```python
from build123d import *

# Parameters (mm, degrees)
SKETCH1_W                  = 38.1
SKETCH1_H                  = 4.365625
BOSS_EXTRUDE1_DEPTH        = 12.7
BOSS_EXTRUDE3_DEPTH        = 12.7
SKETCH8_R                  = 2.1828125
CUT_EXTRUDE1_DEPTH         = 30.170285502
SKETCH11_R                 = 2.1828125
CUT_EXTRUDE2_DEPTH         = 30.170285502
FILLET1_R                  = 3.175
FILLET2_R                  = 3.175
F_4_40_TAPPED_HOLE1_D      = 2.2606
BOSS_EXTRUDE4_DEPTH        = 12.7
TAP_DRILL_FOR_10_32_TAP1_D = 4.0386
FILLET3_R                  = 1.27
FILLET4_R                  = 1.27
CHAMFER1_SIZE              = 0.254


with BuildPart() as part:
    # Sketch1 → Boss-Extrude1 (new body)
    with BuildSketch(Plane.XY):
        Polygon((6.35, 5.08), (25.4, 5.08), (25.4, -5.08), (-25.4, -5.08), (-25.4, 5.08), (-6.35, 5.08), align=None)
        Rectangle(SKETCH1_W, SKETCH1_H, mode=Mode.SUBTRACT)
    extrude(amount=BOSS_EXTRUDE1_DEPTH)

    # Sketch7 → Boss-Extrude3 (add)
    with BuildSketch(Plane.XY.offset(12.7)):
        with BuildLine():
            Line((-20.290450061, 5.08), (-13.443924939, 5.08))
            ThreePointArc((-13.443924939, 5.08), (-16.8671875, 6.6675), (-20.290450061, 5.08))
        make_face()
    boss_extrude3 = extrude(amount=-BOSS_EXTRUDE3_DEPTH)

    # Sketch8 → Cut-Extrude1 (cut, through all)
    with BuildSketch(Plane.XY.offset(12.7)):
        with Locations((-16.8671875, 2.1828125)):
            Circle(SKETCH8_R)
    cut_extrude1 = extrude(amount=-CUT_EXTRUDE1_DEPTH, mode=Mode.SUBTRACT)

    # Sketch11 → Cut-Extrude2 (cut, through all)
    with BuildSketch(Plane.XY.offset(12.7)):
        with Locations((-17.159628923, -1.09140625)):
            Circle(SKETCH11_R)
    cut_extrude2 = extrude(amount=-CUT_EXTRUDE2_DEPTH, mode=Mode.SUBTRACT)

    # Fillet1
    fillet1_edges = [part.edges().sort_by_distance(p)[0] for p in [
        (-13.443924939, 5.08, 6.35),
        (-20.290450061, 5.08, 6.35),
    ]]
    fillet(fillet1_edges, radius=FILLET1_R)

    # Mirror1: Cut-Extrude1, Cut-Extrude2 across plane
    add(cut_extrude1.mirror(Plane(origin=(0, 0, 0), x_dir=(0, 0, 1), z_dir=(1, 0, 0))), mode=Mode.SUBTRACT)
    add(cut_extrude2.mirror(Plane(origin=(0, 0, 0), x_dir=(0, 0, 1), z_dir=(1, 0, 0))), mode=Mode.SUBTRACT)

    # Mirror2: Boss-Extrude3 across plane
    add(boss_extrude3.mirror(Plane(origin=(0, 0, 0), x_dir=(0, 0, 1), z_dir=(1, 0, 0))))

    # Fillet2
    fillet2_edges = [part.edges().sort_by_distance(p)[0] for p in [
        (13.443924939, 5.08, 6.35),
        (20.290450061, 5.08, 6.35),
    ]]
    fillet(fillet2_edges, radius=FILLET2_R)

    # #4-40 Tapped Hole1 (through all)
    with Locations(Plane(origin=(0, -5.08, 0), x_dir=(-1, 0, 0), z_dir=(0, -1, 0))):
        with Locations((22.225, -6.35), (-22.225, -6.35)):
            Hole(F_4_40_TAPPED_HOLE1_D / 2)

    # Sketch10 → Boss-Extrude4 (add)
    with BuildSketch(Plane.XY.offset(12.7)):
        with BuildLine():
            Line((-10.894095156, 5.08), (10.894095156, 5.08))
            ThreePointArc((10.894095156, 5.08), (7.889019146, 5.746209312), (5.447047578, 7.62))
            ThreePointArc((5.447047578, 7.62), (0, 10.16), (-5.447047578, 7.62))
            ThreePointArc((-5.447047578, 7.62), (-7.889019146, 5.746209312), (-10.894095156, 5.08))
        make_face()
    extrude(amount=-BOSS_EXTRUDE4_DEPTH)

    # Tap Drill for #10-32 Tap1 (through all)
    with Locations(Plane.XY.offset(12.7)):
        with Locations((0, 6.17140625)):
            Hole(TAP_DRILL_FOR_10_32_TAP1_D / 2)

    # Fillet3
    fillet3_edges = [part.edges().sort_by_distance(p)[0] for p in [
        (-14.684375, 2.1828125, 6.35),
        (-15.269257847, -2.1828125, 6.35),
        (-19.05, 0, 6.35),
        (14.684375, 2.1828125, 6.35),
        (19.05, 0, 6.35),
        (15.269257847, -2.1828125, 6.35),
    ]]
    fillet(fillet3_edges, radius=FILLET3_R)

    # Fillet4
    fillet4_edges = [part.edges().sort_by_distance(p)[0] for p in [
        (-25.4, 5.08, 6.35),
        (25.4, 5.08, 6.35),
    ]]
    fillet(fillet4_edges, radius=FILLET4_R)

    # Chamfer1
    chamfer1_edges = [part.edges().sort_by_distance(p)[0] for p in [
        (-18.362829894, -2.912663462, 0),
        (0, -2.1828125, 0),
        (18.362829894, -2.912663462, 0),
        (19.05, 1.241039162, 0),
        (17.275850124, 4.327029203, 0),
        (0, 2.1828125, 0),
        (-17.275850124, 4.327029203, 0),
        (-14.370442252, 2.402538589, 0),
        (14.370442252, 2.402538589, 0),
        (-15.14545512, -2.287485231, 0),
        (15.14545512, -2.287485231, 0),
        (19.077182057, 0.037916326, 0),
        (-19.077182057, 0.037916326, 0),
        (-19.05, 1.241039162, 0),
    ]]
    chamfer(chamfer1_edges, length=CHAMFER1_SIZE)


solid = part.part
```
Geometry check sheet. Reference: the model listing, model coordinates, mm. A direction names the side the tool comes from. Round coordinates to 2 decimals unless told otherwise and drop trailing zeros. Order: outer loops, then holes, each group sorted by start corner. A loop starts at its lowest first (then second) coordinate and runs counter-clockwise, first axis right, second up. Notation, with made-up numbers: (32.5, -16.5) -> (46.5, -16.5) arc R7 cw to (46.5, -12.5) -> close; hole circle Ø1 at (-19.75, 0). An arc over 180 degrees is marked (long way). Return JSON: item names as keys, results as strings. Group by question number.
Q1. Release check for a two-part mould opening along X. For faces 1 (the cylindrical face through (20.528, 5.244, 6.261)), 2 (the flat face through (12, 5.08, 6)), 3 (the cylindrical face through (-17.234, 4.335, 6.564)), 4 (the flat face through (0, -5.08, 6)) record: released by +X, released by -X, zero draft, split by the parting line, or undercut.
Q2. Section check A-A, the plane y = 1. Record the boundary of the cut face in (x, z) (3 decimals), plus the area to 3 significant figures.
Q3. Tool access check on faces 5 (the flat face through (-12, 5.08, 6)), 6 (the flat face through (0, -2.183, 6)), 7 (the flat face through (-25.4, -1, 6)). Record the directions out of +Z, -Z, +X, -X, +Y, -Y that give a thin tool (end or side, any length) a straight path to the whole face; none if there is none.
Q4. Section check B-B, the plane x = 0. Record the boundary of the cut face in (y, z).
Q5. Section check C-C, the plane z = 10.25. Count the separate pieces of the cut face and the enclosed holes in it, plus the area to 3 significant figures.
Q6. Material ranges on probe 1 along Y at (x, z) = (0, 8.25); probe 2 along X at (y, z) = (2, 6.35); probe 3 along X at (y, z) = (4, 1.5), recorded low to high. Write a range as from..to.
Q7. Gauge pin test, flat ends, axial feed: pin 1 (2 mm diameter, centred on x = 22, z = 9, fed in from +Y); pin 2 (5.5 mm diameter, centred on x = 0, y = 6.17, fed in from +Z); pin 3 (1 mm diameter, centred on y = 6.5, z = 8.5, fed in from +X). Record the tip position at first contact, or that the pin passes through.
Numbers:
{
 "1": {"face 1": "released by +X", "face 2": "undercut", "face 3": "undercut", "face 4": "zero draft"},
 "2": {"outline": "(-25.4, 0) -> (-19.304, 0) -> (-19.05, 0.254) -> (-19.05, 12.7) -> (-25.4, 12.7) -> close; (19.05, 0.254) -> (19.304, 0) -> (25.4, 0) -> (25.4, 12.7) -> (19.05, 12.7) -> close; hole circle Ø2.261 at (-22.225, 6.35); hole circle Ø2.261 at (22.225, 6.35)", "area": "153 mm^2"},
 "3": {"face 5": "+Z, -Z, +Y", "face 6": "+Z, -Z", "face 7": "+Z, -Z, -X, +Y, -Y"},
 "4": {"outline": "(-5.08, 0) -> (-2.44, 0) -> (-2.18, 0.25) -> (-2.18, 12.7) -> (-5.08, 12.7) -> close; (2.18, 0.25) -> (2.44, 0) -> (4.15, 0) -> (4.15, 12.7) -> (2.18, 12.7) -> close; (8.19, 0) -> (10.16, 0) -> (10.16, 12.7) -> (8.19, 12.7) -> close"},
 "5": {"separate pieces": "1", "enclosed holes": "2", "area": "385 mm^2"},
 "6": {"probe 1": "-5.08..-2.18, 2.18..4.15, 8.19..10.16", "probe 2": "-25.4..-23.36, -21.09..-19.05, 19.05..21.09, 23.36..25.4", "probe 3": "-25.39..-18.08, -15.66..15.66, 18.08..25.39"},
 "7": {"pin 1": "y = 5.13", "pin 2": "z = 12.7", "pin 3": "x = 19.22"}
}
